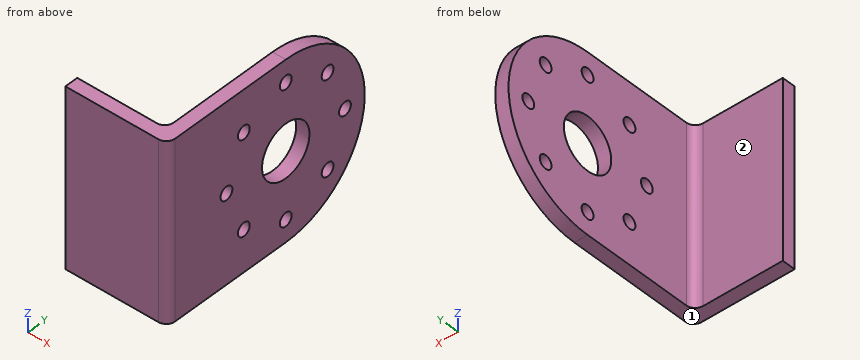
from build123d import *

# Parameters (mm, degrees)
BOSS_EXTRUDE1_OUTLINE_R   = 1.5
BOSS_EXTRUDE1_OUTLINE_R_2 = 6
BOSS_EXTRUDE1_DEPTH       = 3
SKETCH2_W                 = 40
SKETCH2_H                 = 3
BOSS_EXTRUDE2_DEPTH       = 20
FILLET1_R                 = 2
FILLET2_R                 = 2


# Read off the part's stored shape, not the designer's step: Boss-Extrude1
with BuildPart() as part:
    # Boss-Extrude1 outline → Boss-Extrude1 (new body)
    with BuildSketch(Plane(origin=(0, 0, 0), x_dir=(0, 0, -1), z_dir=(1, 0, 0))):
        with BuildLine():
            Line((20, -30), (20, 0))
            ThreePointArc((20, 0), (0, 20), (-20, 0))
            Line((-20, 0), (-20, -30))
            Line((-20, -30), (20, -30))
        make_face()
        with Locations((-10.606601718, -10.606601718)):
            Circle(BOSS_EXTRUDE1_OUTLINE_R, mode=Mode.SUBTRACT)
        with Locations((0, -15)):
            Circle(BOSS_EXTRUDE1_OUTLINE_R, mode=Mode.SUBTRACT)
        with Locations((10.606601718, -10.606601718)):
            Circle(BOSS_EXTRUDE1_OUTLINE_R, mode=Mode.SUBTRACT)
        with Locations((-15, 0)):
            Circle(BOSS_EXTRUDE1_OUTLINE_R, mode=Mode.SUBTRACT)
        with Locations((-10.606601718, 10.606601718)):
            Circle(BOSS_EXTRUDE1_OUTLINE_R, mode=Mode.SUBTRACT)
        Circle(BOSS_EXTRUDE1_OUTLINE_R_2, mode=Mode.SUBTRACT)
        with Locations((15, 0)):
            Circle(BOSS_EXTRUDE1_OUTLINE_R, mode=Mode.SUBTRACT)
        with Locations((0, 15)):
            Circle(BOSS_EXTRUDE1_OUTLINE_R, mode=Mode.SUBTRACT)
        with Locations((10.606601718, 10.606601718)):
            Circle(BOSS_EXTRUDE1_OUTLINE_R, mode=Mode.SUBTRACT)
    extrude(amount=BOSS_EXTRUDE1_DEPTH)

    # Sketch2 → Boss-Extrude2 (add)
    with BuildSketch(Plane.ZY):
        with Locations((0, -28.5)):
            Rectangle(SKETCH2_W, SKETCH2_H)
    extrude(amount=BOSS_EXTRUDE2_DEPTH)

    # Fillet1
    fillet1_edges = [part.edges().sort_by_distance(p)[0] for p in [
        (3, -30, 0),
    ]]
    fillet(fillet1_edges, radius=FILLET1_R)

    # Fillet2
    fillet2_edges = [part.edges().sort_by_distance(p)[0] for p in [
        (0, -27, 0),
    ]]
    fillet(fillet2_edges, radius=FILLET2_R)


solid = part.part
Can you work these out from the model? Positions are in its coordinate system, mm. Face numbers are marked on the shaded views. A direction names the side the tool comes from. Give positions to 0.01 mm unless a question says otherwise; leave off trailing zeros. Loops run counter-clockwise (first coordinate to the right, second up) from the corner with the lowest first, then second, coordinate; pieces in that order, holes last. Notation, with made-up numbers: (45.25, 24.25) -> (94.25, 24.25) arc R26 cw to (94.25, 61.25) -> close; hole circle Ø9 at (3, -39). An arc over 180 degrees is marked (long way). Return JSON: item names as keys, results as strings.
Q1. I want a section at B-B, the plane z = -5. List the corners of the cut face in (x, y) for me.
Checks:
{"outline": "(-20, -30) -> (1, -30) arc R2 ccw to (3, -28) -> (3, -3.32) -> (0, -3.32) -> (0, -25) arc R2 cw to (-2, -27) -> (-20, -27) -> close; (0, 3.32) -> (3, 3.32) -> (3, 19.36) -> (0, 19.36) -> close"}
Q2. On a 3-axis mill with a long thin cutter (end or side, diameter ignored), from which of +Z, -Z, +X, -X, +Y, -Y can I reach the whole of each face in a straight line? I mean the marked faces 1 and 2. Say none if no direction works.
Checks:
{"face 1": "-Z, +X, -X, +Y, -Y", "face 2": "+Z, -Z, -X, +Y"}
Q3. I want a section at A-A, the plane y = -15. List the corners of the cut face in (x, z) for me.
Checks:
{"outline": "(0, -20) -> (3, -20) -> (3, -1.5) -> (0, -1.5) -> close; (0, 1.5) -> (3, 1.5) -> (3, 20) -> (0, 20) -> close"}
Q4. I need wall thicknesses on probe 1 along Y at (x, z) = (0.5, 0); probe 2 along Y at (x, z) = (2.2, 0); probe 3 along X at (y, z) = (-9, -6). Which ranges of each line are inside material? Lowest first, please.
Checks:
{"probe 1": "y = -30 to -16.5, -13.5 to -6, 6 to 13.5, 16.5 to 20", "probe 2": "y = -29.6 to -16.5, -13.5 to -6, 6 to 13.5, 16.5 to 20", "probe 3": "x = 0 to 3"}
Q5. I want a section at D-D, the plane y = 10. List the corners of the cut face in (x, z) for me.
Checks:
{"outline": "(0, -17.32) -> (3, -17.32) -> (3, -11.98) -> (0, -11.98) -> close; (0, -9.23) -> (3, -9.23) -> (3, 9.23) -> (0, 9.23) -> close; (0, 11.98) -> (3, 11.98) -> (3, 17.32) -> (0, 17.32) -> close"}
Q6. For pin 1 Ø2.5 at (y, z) = (0, 15) entering from +X; pin 2 Ø8 at (y, z) = (-16.5, -12) entering from -X; pin 3 Ø3 at (x, z) = (-1, 7.5) entering from +Y; pin 4 Ø5.5 at (x, z) = (-12.5, 5.5) entering from +Y, each with a flat end and sliding along its axis, tell me the tip position at first contact or that it passes through.
Checks:
{"pin 1": "passes through", "pin 2": "stops at x = 0", "pin 3": "stops at y = 18.95", "pin 4": "stops at y = -27"}
Q7. I want a section at C-C, the plane z = -0.5. List the corners of the cut face in (x, y) for me, then the cut area to 3 significant figures.
Checks:
{"outline": "(-20, -30) -> (1, -30) arc R2 ccw to (3, -28) -> (3, -16.41) -> (0, -16.41) -> (0, -25) arc R2 cw to (-2, -27) -> (-20, -27) -> close; (0, -13.59) -> (3, -13.59) -> (3, -5.98) -> (0, -5.98) -> close; (0, 5.98) -> (3, 5.98) -> (3, 13.59) -> (0, 13.59) -> close; (0, 16.41) -> (3, 16.41) -> (3, 19.99) -> (0, 19.99) -> close", "area": "157 mm2"}
